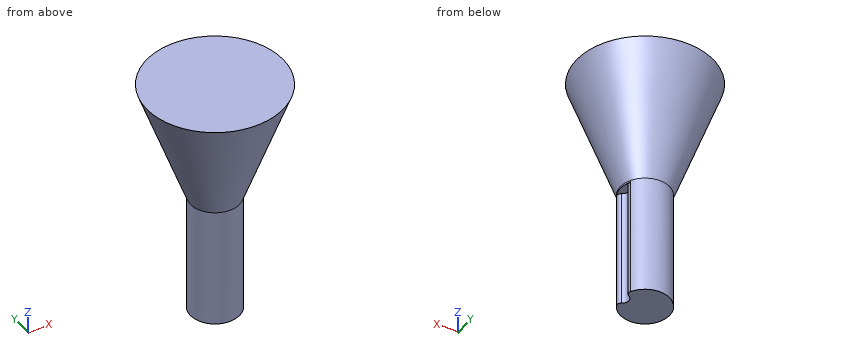
from build123d import *
from build123d import SkipClean  # not in build123d's __all__

# Parameters (mm, degrees)
F1_DEPTH = 12.7
F2_R     = 2.6
F3_DEPTH = 12.7
F3_TAPER = -20
F6_DEPTH = 0.2


with BuildPart() as f1:
    # F0 (on Top) → F1 (new body)
    with BuildSketch(Plane.XY):
        with BuildLine():
            ThreePointArc((2.0857885615, 0.6255167239), (2.315451032, 0.8961675136), (2.2801491146, 1.2493678462))
            ThreePointArc((2.2801491146, 1.2493678462), (-2.6, 0), (2.2801491146, -1.2493678462))
            ThreePointArc((2.2801491146, -1.2493678462), (2.315451032, -0.8961675136), (2.0857885615, -0.6255167239))
            ThreePointArc((2.0857885615, -0.6255167239), (1.7, 0), (2.0857885615, 0.6255167239))
        make_face()
    extrude(amount=-F1_DEPTH)

    # F2 (on Top) → F3 (join)
    with BuildSketch(Plane.XY):
        Circle(F2_R)
    extrude(amount=F3_DEPTH, taper=F3_TAPER)

    # F5 (on face) → F6 (join)
    with BuildSketch(Plane(origin=(0, 0, 0), x_dir=(1, 0, 0), z_dir=(0, 0, -1))):
        with BuildLine():
            ThreePointArc((2.2801491146, 1.2493678462), (2.315451032, 0.8961675136), (2.0857885615, 0.6255167239))
            ThreePointArc((2.0857885615, 0.6255167239), (1.7, 0), (2.0857885615, -0.6255167239))
            ThreePointArc((2.0857885615, -0.6255167239), (2.315451032, -0.8961675136), (2.2801491146, -1.2493678462))
            ThreePointArc((2.2801491146, -1.2493678462), (2.6, 0), (2.2801491146, 1.2493678462))
        make_face()
    with SkipClean():  # cleaning this boolean's faces spoils the solid; the shape is the same uncleaned
        extrude(amount=F6_DEPTH)


solid = f1.part
Geometry check sheet. Reference: the model listing, model coordinates, mm. Round coordinates to 2 decimals unless told otherwise and drop trailing zeros. Write each loop counter-clockwise with the first axis right and the second up, starting at its lowest first coordinate (ties: lowest second). Pieces come first, ordered by that corner, then holes. Notation, with made-up numbers: (74, 77) -> (132, 77) arc R36 cw to (132, 111) -> close; hole circle Ø9 at (65, 10.25). An arc over 180 degrees is marked (long way). One line per item, written item: value. Start each with the question number.
(1) Cross-section at B-B, the plane z = -2.75. Record the cut outline in (x, y).
(2) Go/stop test with a flat-tipped pin: pin 1 Ø5 at (y, z) = (4, -10) entering from +X. Record where the tip stops, or that it passes through.
(3) Cross-section at C-C, the plane z = 4.75. Record the cut outline in (x, y), and give its area (3 significant figures).
(4) Scan lines: line 1 (Z direction, x = 2.5, y = 4.5); line 2 (X direction, y = -0.5, z = 10.5); line 3 (Y direction, x = -1.75, z = 5.25). Record each from-to range of solid material in increasing order. Write a range as [from, to].
(5) Cross-section at A-A, the plane x = 0. Record the cut outline in (y, z), and give its area (3 significant figures).
Answer:
1. outline: (2.09, -0.63) arc R0.7 cw to (2.09, 0.63) arc R0.45 ccw to (2.28, 1.25) arc R2.6 ccw (long way) to (2.28, -1.25) arc R0.45 ccw to start
2. pin 1: x = 2.12
3. outline: circle Ø8.66 at (0, 0)
3. area: 58.9 mm²
4. line 1: [7, 12.7]
4. line 2: [-6.4, 6.4]
4. line 3: [-4.16, 4.16]
5. outline: (-7.22, 12.7) -> (-2.6, 0) -> (-2.6, -12.7) -> (2.6, -12.7) -> (2.6, 0) -> (7.22, 12.7) -> close
5. area: 191 mm²
